Part print with two shaded views. Sizes in mm from the minimum x, y, z corner. A direction names the side the tool comes from. Give positions to 0.01 mm unless a question says otherwise; leave off trailing zeros. Order: outer loops, then holes, each group sorted by start corner. A loop starts at its lowest first (then second) coordinate and runs counter-clockwise, first axis right, second up. Notation, with made-up numbers: M 31,-18 L 50,-18 A29 ccw 50,21 Z; hole C 12,68 d4. An arc over 180 degrees is marked long. Return JSON: item names as keys, results as strings.
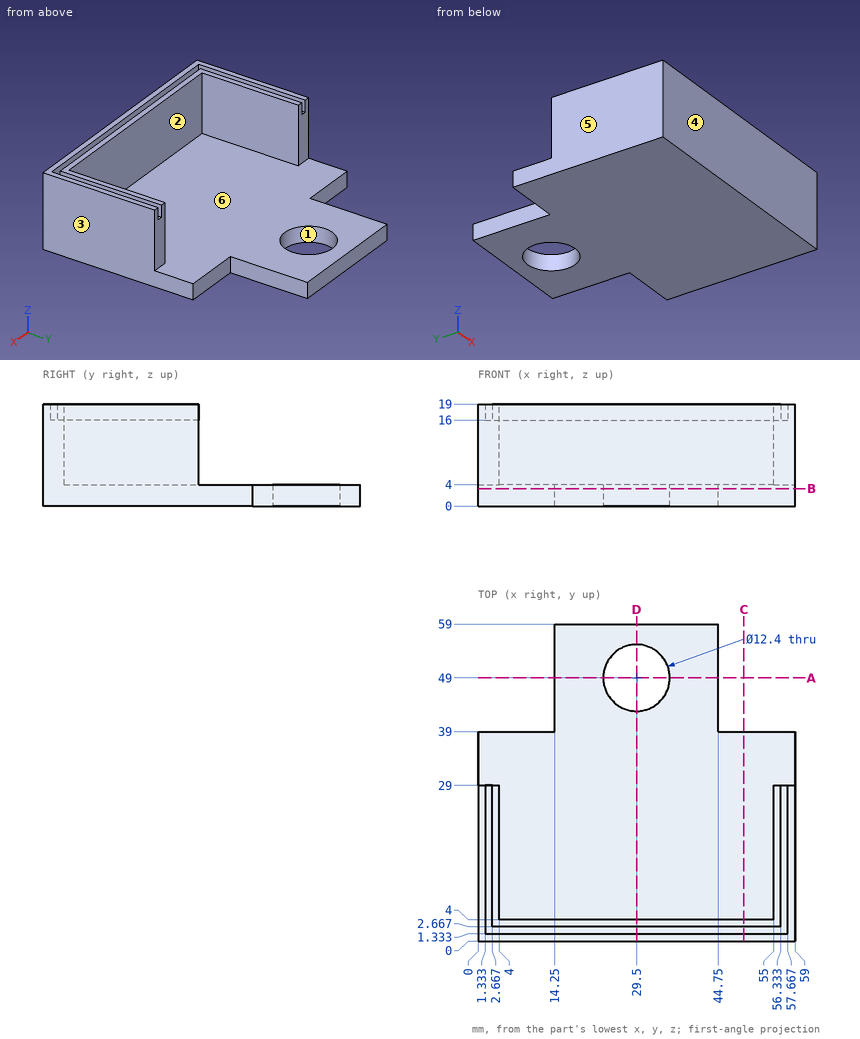
Q1. Band-saw the part on B-B (z = 3.25). Give the cut face in (x, y), then the cut area to 3 significant figures.
Established:
{"outline": "M 0,0 L 59,0 L 59,39 L 44.75,39 L 44.75,59 L 14.25,59 L 14.25,39 L 0,39 Z; hole C 29.5,49 d12.4", "area": "2,790 mm²"}
Q2. Pin check, flat tips, straight feed: pin 1 (4.5 mm diameter, centred on y = 44.5, z = 3, fed in from +X); pin 2 (2.5 mm diameter, centred on y = 13.5, z = 17.5, fed in from -X); pin 3 (4.5 mm diameter, centred on x = 20, z = 8, fed in from +Y); pin 4 (2 mm diameter, centred on x = 54.5, z = 1.5, fed in from +Y). Stop position of each tip, or through.
Established:
{"pin 1": "stops at x = 44.75", "pin 2": "stops at x = 0", "pin 3": "stops at y = 4", "pin 4": "stops at y = 39"}
Q3. Band-saw the part on C-C (x = 49.5). Give the cut face in (y, z).
Established:
{"outline": "M 0,0 L 39,0 L 39,4 L 4,4 L 4,19 L 2.67,19 L 2.67,16 L 1.33,16 L 1.33,19 L 0,19 Z"}
Q4. Band-saw the part on D-D (x = 29.5). Give the cut face in (y, z).
Established:
{"outline": "M 0,0 L 42.8,0 L 42.8,4 L 4,4 L 4,19 L 2.67,19 L 2.67,16 L 1.33,16 L 1.33,19 L 0,19 Z; M 55.2,0 L 59,0 L 59,4 L 55.2,4 Z"}
Q5. Two-plate mould, pull along X, no slides. Class the marked faces 3, 4, 5 and 6: +X half, -X half, draft (parallel to the pull), parting line (faces both ways), or undercut.
Established:
{"face 3": "+X half", "face 4": "draft", "face 5": "-X half", "face 6": "undercut"}
Q6. Band-saw the part on A-A (y = 49). Give the cut face in (x, z).
Established:
{"outline": "M 14.25,0 L 23.3,0 L 23.3,4 L 14.25,4 Z; M 35.7,0 L 44.75,0 L 44.75,4 L 35.7,4 Z"}
Q7. Probe line 1 along X through (y, z) = (9, 16.5); line 2 along Y through (x, z) = (29.5, 2.5); line 3 along X through (y, z) = (7.5, 7.25). List the from-to ranges inside material, lowest first.
Established:
{"line 1": "x = 0 to 1.33, 2.67 to 4, 55 to 56.33, 57.67 to 59", "line 2": "y = 0 to 42.8, 55.2 to 59", "line 3": "x = 0 to 4, 55 to 59"}
Q8. 3-axis set-ups, long thin cutter, end or side, ignore diameter. For the marked faces 1 and 2: which of +Z, -Z, +X, -X, +Y, -Y reach the whole face in a straight line?
Established:
{"face 1": "+Z, -Z", "face 2": "+Z, +Y"}
